Could you check a few things on this drawing? It's one solid part, dimensions in mm from its lowest x, y, z. A direction names the side the tool comes from. Round coordinates to 2 decimals unless told otherwise and drop trailing zeros. Write each loop counter-clockwise with the first axis right and the second up, starting at its lowest first coordinate (ties: lowest second). Pieces come first, ordered by that corner, then holes. Notation, with made-up numbers: (35.25, 89) -> (78.25, 89) arc R21 ccw to (78.25, 97) -> close; hole circle Ø8 at (18, -38). An arc over 180 degrees is marked (long way). Answer in a Markdown table with one row per item.
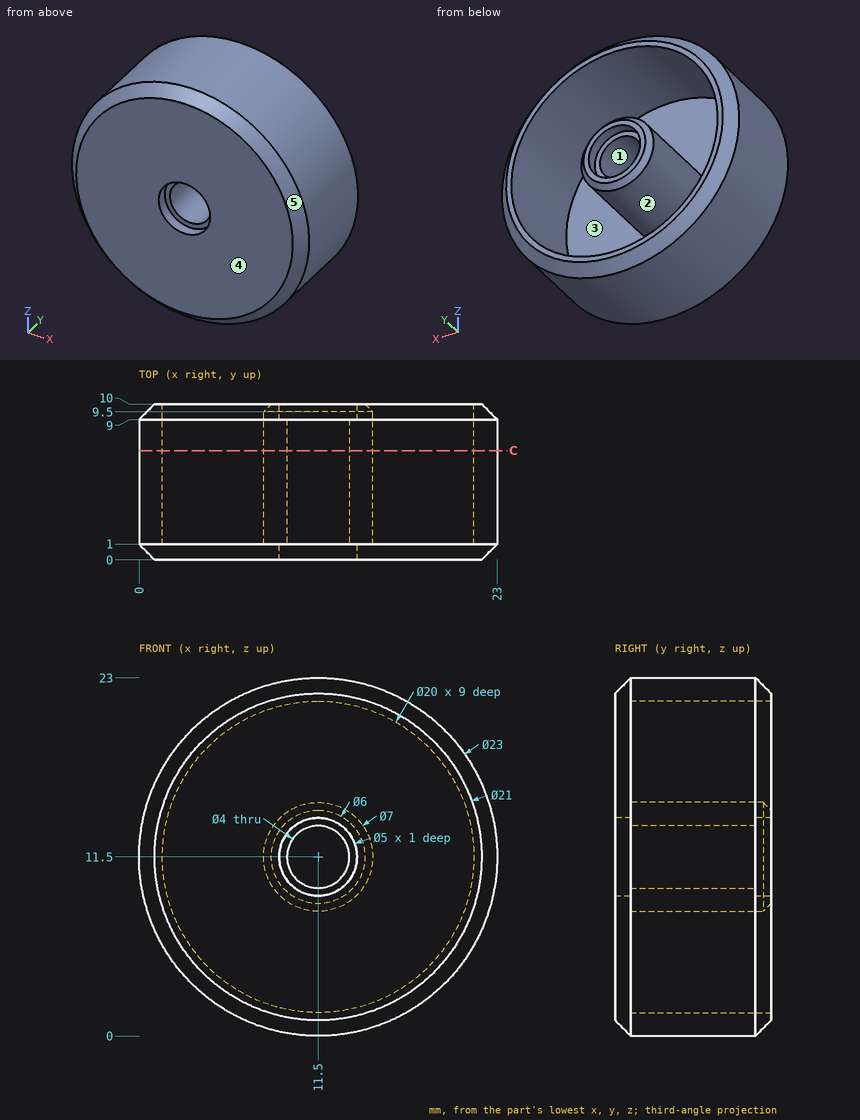
1) Thinking about a two-plate mould opening in X: for the marked faces 3, 4 and 5, which applies, +X half, -X half, draft (parallel to the pull), parting line (faces both ways), or undercut?
Findings:
| item | result |
|---|---|
| face 3 | undercut |
| face 4 | draft |
| face 5 | parting line |
2) Imagine slicing it at C-C, the plane y = 7. Please give me the cut outline in (x, z), plus the area to 3 significant figures.
Findings:
| item | result |
|---|---|
| outline | circle Ø23 at (11.5, 11.5); circle Ø7 at (11.5, 11.5); hole circle Ø20 at (11.5, 11.5); hole circle Ø4 at (11.5, 11.5) |
| area | 127 mm^2 |
3) For pin 1 (3 mm diameter, centred on x = 6.5, z = 14.5, fed in from +Y); pin 2 (12 mm diameter, centred on x = 9.5, z = 12, fed in from -Y); pin 3 (1 mm diameter, centred on y = 1, z = 16, fed in from -X); pin 4 (2.5 mm diameter, centred on x = 11.5, z = 11.5, fed in from -Y), each with a flat end and sliding along its axis, tell me the tip position at first contact or that it passes through.
Findings:
| item | result |
|---|---|
| pin 1 | stops at y = 1 |
| pin 2 | stops at y = 0 |
| pin 3 | stops at x = 0.72 |
| pin 4 | passes through |
4) Please list where these lines run through material, in increasing order: line 1 (X direction, y = 5.75, z = 11.5); line 2 (X direction, y = 9.3, z = 11.5); line 3 (Z direction, x = 14, y = 8.5).
Findings:
| item | result |
|---|---|
| line 1 | x = 0 to 1.5, 8 to 9.5, 13.5 to 15, 21.5 to 23 |
| line 2 | x = 0.3 to 1.5, 8 to 9, 14 to 15, 21.5 to 22.7 |
| line 3 | z = 0.28 to 1.82, 9.05 to 13.95, 21.18 to 22.72 |
5) For the marked faces 1 and 2, which set-ups out of +Z, -Z, +X, -X, +Y, -Y let a thin tool reach every point of the face, with its end or its side?
Findings:
| item | result |
|---|---|
| face 1 | +Y, -Y |
| face 2 | +Y |
